from build123d import *

# Parameters (mm, degrees)
PAD021_DEPTH                  = 40.5
POCKET064_DEPTH               = 6
PAD021_MIRRORED041_2_DEPTH    = 40.5
POCKET064_MIRRORED041_2_DEPTH = 6
PAD022_DEPTH                  = 2
PAD022_MIRRORED032_2_DEPTH    = 2
POCKET055_DEPTH               = 30.5
PAD018_DEPTH                  = 19.5
PAD018_FACE36_W               = 39
PAD018_FACE36_H               = 1.2
POCKET061_DEPTH               = 0.2
CHAMFER032_SIZE               = 0.5
CHAMFER030_SIZE               = 1
CHAMFER027_SIZE               = 0.2999
POCKET058_DEPTH               = 10
SKETCH064_W                   = 9.4
SKETCH064_H                   = 50
POCKET070_DEPTH               = 15
POCKET059_DEPTH               = 5
POCKET069_DEPTH               = 10
POCKET062_DEPTH               = 10
POCKET051_DEPTH               = 10
POCKET067_DEPTH               = 10
POCKET054_DEPTH               = 10


with BuildPart() as part:
    # Sketch081 (on DatumPlane) → Pad021 (new body)
    with BuildSketch(Plane.XY.offset(50)):
        with BuildLine():
            ThreePointArc((-47.2, 27.2), (-50.735534, 25.735534), (-52.2, 22.2))
            Line((-52.2, 0), (-52.2, 22.2))
            Line((-50.2, 0), (-52.2, 0))
            Line((-50.2, 22.2), (-50.2, 0))
            ThreePointArc((-47.2, 25.2), (-49.32132, 24.32132), (-50.2, 22.2))
            Line((0, 25.2), (-47.2, 25.2))
            Line((0, 27.2), (0, 25.2))
            Line((-47.2, 27.2), (0, 27.2))
        make_face()
    pad021 = extrude(amount=-PAD021_DEPTH)

    # Sketch080 (on Face10 of Pad021) → Pocket064 (cut)
    with BuildSketch(Plane(origin=(0, 0, 9.5), x_dir=(1, 0, 0), z_dir=(0, 0, -1))):
        with BuildLine():
            ThreePointArc((-50.2, -22.2), (-49.32132, -24.32132), (-47.2, -25.2))
            Line((-47.2, -25.2), (0, -25.2))
            Line((0, -25.2), (0, -26.3))
            Line((0, -26.3), (-47.2, -26.3))
            ThreePointArc((-51.3, -22.2), (-50.099138, -25.099138), (-47.2, -26.3))
            Line((-51.3, 0), (-51.3, -22.2))
            Line((-50.2, 0), (-51.3, 0))
            Line((-50.2, -22.2), (-50.2, 0))
        make_face()
    pocket064 = extrude(amount=-POCKET064_DEPTH, mode=Mode.SUBTRACT)

    # Sketch081 Mirrored041 2 → Pad021 Mirrored041 2 (add)
    with BuildSketch(Plane(origin=(0, 0, 50), x_dir=(-1, 0, 0), z_dir=(0, 0, -1))):
        with BuildLine():
            ThreePointArc((-47.2, 27.2), (-50.735534, 25.735534), (-52.2, 22.2))
            Line((-52.2, 0), (-52.2, 22.2))
            Line((-50.2, 0), (-52.2, 0))
            Line((-50.2, 22.2), (-50.2, 0))
            ThreePointArc((-47.2, 25.2), (-49.32132, 24.32132), (-50.2, 22.2))
            Line((0, 25.2), (-47.2, 25.2))
            Line((0, 27.2), (0, 25.2))
            Line((-47.2, 27.2), (0, 27.2))
        make_face()
    pad021_mirrored041_2 = extrude(amount=PAD021_MIRRORED041_2_DEPTH)

    # Sketch080 Mirrored041 2 → Pocket064 Mirrored041 2 (cut)
    with BuildSketch(Plane(origin=(0, 0, 9.5), x_dir=(-1, 0, 0), z_dir=(0, 0, 1))):
        with BuildLine():
            ThreePointArc((-50.2, -22.2), (-49.32132, -24.32132), (-47.2, -25.2))
            Line((-47.2, -25.2), (0, -25.2))
            Line((0, -25.2), (0, -26.3))
            Line((0, -26.3), (-47.2, -26.3))
            ThreePointArc((-51.3, -22.2), (-50.099138, -25.099138), (-47.2, -26.3))
            Line((-51.3, 0), (-51.3, -22.2))
            Line((-50.2, 0), (-51.3, 0))
            Line((-50.2, -22.2), (-50.2, 0))
        make_face()
    pocket064_mirrored041_2 = extrude(amount=POCKET064_MIRRORED041_2_DEPTH, mode=Mode.SUBTRACT)

    # Mirrored036: Pad021, Pocket064, Pad021 Mirrored041 2, Pocket064 Mirrored041 2 across Sketch081 H_Axis
    add(pad021.mirror(Plane(origin=(0, 0, 50), x_dir=(0, 0, 1), z_dir=(0, 1, 0))))
    add(pocket064.mirror(Plane(origin=(0, 0, 50), x_dir=(0, 0, 1), z_dir=(0, 1, 0))), mode=Mode.SUBTRACT)
    add(pad021_mirrored041_2.mirror(Plane(origin=(0, 0, 50), x_dir=(0, 0, 1), z_dir=(0, 1, 0))))
    add(pocket064_mirrored041_2.mirror(Plane(origin=(0, 0, 50), x_dir=(0, 0, 1), z_dir=(0, 1, 0))), mode=Mode.SUBTRACT)

    # Sketch058 (on DatumPlane) → Pad022 (join)
    with BuildSketch(Plane.XY.offset(50)):
        with BuildLine():
            ThreePointArc((-47.2, 25.2), (-49.32132, 24.32132), (-50.2, 22.2))
            Line((-50.2, 22.2), (-50.2, 0))
            Line((-50.2, 0), (0, 0))
            Line((0, 0), (0, 25.2))
            Line((0, 25.2), (-47.2, 25.2))
        make_face()
    pad022 = extrude(amount=-PAD022_DEPTH)

    # Sketch058 Mirrored032 2 → Pad022 Mirrored032 2 (add)
    with BuildSketch(Plane(origin=(0, 0, 50), x_dir=(-1, 0, 0), z_dir=(0, 0, -1))):
        with BuildLine():
            ThreePointArc((-47.2, 25.2), (-49.32132, 24.32132), (-50.2, 22.2))
            Line((-50.2, 22.2), (-50.2, 0))
            Line((-50.2, 0), (0, 0))
            Line((0, 0), (0, 25.2))
            Line((0, 25.2), (-47.2, 25.2))
        make_face()
    pad022_mirrored032_2 = extrude(amount=PAD022_MIRRORED032_2_DEPTH)

    # Mirrored039: Pad022, Pad022 Mirrored032 2 across Sketch058 H_Axis
    add(pad022.mirror(Plane(origin=(0, 0, 50), x_dir=(0, 0, 1), z_dir=(0, 1, 0))))
    add(pad022_mirrored032_2.mirror(Plane(origin=(0, 0, 50), x_dir=(0, 0, 1), z_dir=(0, 1, 0))))

    # Sketch067 → Pocket055 (cut, symmetric)
    with BuildSketch(Plane.YZ):
        with BuildLine():
            ThreePointArc((-26.1, 12.9), (-26.7, 12.3), (-26.1, 11.7))
            Line((-26.1, 12.9), (-26.1, 11.7))
        make_face()
    pocket055 = extrude(amount=POCKET055_DEPTH, both=True, mode=Mode.SUBTRACT)

    # Sketch067 → Pad018 (join, symmetric)
    with BuildSketch(Plane.YZ):
        with BuildLine():
            ThreePointArc((-26.1, 12.9), (-26.7, 12.3), (-26.1, 11.7))
            Line((-26.1, 12.9), (-26.1, 11.7))
        make_face()
    pad018 = extrude(amount=PAD018_DEPTH, both=True)

    # Pad018 Face36 → Pocket061 (cut)
    with BuildSketch(Plane(origin=(0, -26.1, 12.3), x_dir=(1, 0, 0), z_dir=(0, 1, 0))):
        Rectangle(PAD018_FACE36_W, PAD018_FACE36_H)
    pocket061 = extrude(amount=-POCKET061_DEPTH, mode=Mode.SUBTRACT)

    # Mirrored040: Pocket055, Pad018, Pocket061 across Sketch067 V_Axis
    add(pocket055.mirror(Plane(origin=(0, 0, 0), x_dir=(1, 0, 0), z_dir=(0, 1, 0))), mode=Mode.SUBTRACT)
    add(pad018.mirror(Plane(origin=(0, 0, 0), x_dir=(1, 0, 0), z_dir=(0, 1, 0))))
    add(pocket061.mirror(Plane(origin=(0, 0, 0), x_dir=(1, 0, 0), z_dir=(0, 1, 0))), mode=Mode.SUBTRACT)

    # Chamfer032
    chamfer032_edges = [part.edges().sort_by_distance(p)[0] for p in [
        (0, -27.2, 9.5),
    ]]
    chamfer(chamfer032_edges, length=CHAMFER032_SIZE)

    # Chamfer030
    chamfer030_edges = [part.edges().sort_by_distance(p)[0] for p in [
        (0, -27.2, 50),
    ]]
    chamfer(chamfer030_edges, length=CHAMFER030_SIZE)

    # Chamfer027
    chamfer027_edges = [part.edges().sort_by_distance(p)[0] for p in [
        (50.2, 0, 48),
    ]]
    chamfer(chamfer027_edges, length=CHAMFER027_SIZE)

    # Sketch079 (on DatumPlane) → Pocket058 (cut)
    with BuildSketch(Plane.YZ.offset(52.2)):
        Polygon((-7.2, 7.6), (-7.2, 15.6), (-12.1, 15.6), (-12.1, 18.1), (-14.1, 18.1), (-14.1, 15.6), (-17.8, 15.6), (-17.8, 7.6), (-17.8, 2.6), (-7.2, 2.6), align=None)
    extrude(amount=-POCKET058_DEPTH, mode=Mode.SUBTRACT)

    # Sketch064 (on DatumPlane) → Pocket070 (cut)
    with BuildSketch(Plane.YZ.offset(52.2)):
        with Locations((0, -6)):
            Rectangle(SKETCH064_W, SKETCH064_H)
    extrude(amount=-POCKET070_DEPTH, mode=Mode.SUBTRACT)

    # Sketch065 (on DatumPlane) → Pocket059 (cut)
    with BuildSketch(Plane.YZ.offset(52.2)):
        with BuildLine():
            Line((7.9, -40.25), (7.9, 9.75))
            ThreePointArc((9.15, 11), (8.266117, 10.633883), (7.9, 9.75))
            Line((9.15, 11), (15.85, 11))
            ThreePointArc((17.1, 9.75), (16.733883, 10.633883), (15.85, 11))
            Line((17.1, 9.75), (17.1, -40.25))
            Line((7.9, -40.25), (17.1, -40.25))
        make_face()
    extrude(amount=-POCKET059_DEPTH, mode=Mode.SUBTRACT)

    # Sketch078 (on DatumPlane) → Pocket069 (cut)
    with BuildSketch(Plane(origin=(-52.2, 0, 0), x_dir=(0, -1, 0), z_dir=(-1, 0, 0))):
        Polygon((-15.02, 7.6), (-15.02, 15.6), (-20.32, 15.6), (-20.32, 18.1), (-22.32, 18.1), (-22.32, 15.6), (-25.62, 15.6), (-25.62, 7.6), (-25.62, -42.4), (-15.02, -42.4), align=None)
    extrude(amount=-POCKET069_DEPTH, mode=Mode.SUBTRACT)

    # Sketch075 (on DatumPlane) → Pocket062 (cut)
    with BuildSketch(Plane(origin=(-52.2, 0, 0), x_dir=(0, -1, 0), z_dir=(-1, 0, 0))):
        Polygon((-4.86, 7.6), (-4.86, 15.6), (-10.16, 15.6), (-10.16, 18.1), (-12.16, 18.1), (-12.16, 15.6), (-15.46, 15.6), (-15.46, 7.6), (-15.46, -42.4), (-4.86, -42.4), align=None)
    extrude(amount=-POCKET062_DEPTH, mode=Mode.SUBTRACT)

    # Sketch073 (on DatumPlane) → Pocket051 (cut)
    with BuildSketch(Plane(origin=(-52.2, 0, 0), x_dir=(0, -1, 0), z_dir=(-1, 0, 0))):
        Polygon((5.3, 7.6), (5.3, 15.6), (0, 15.6), (0, 18.1), (-2, 18.1), (-2, 15.6), (-5.3, 15.6), (-5.3, 7.6), (-5.3, -42.4), (5.3, -42.4), align=None)
    extrude(amount=-POCKET051_DEPTH, mode=Mode.SUBTRACT)

    # Sketch077 (on DatumPlane) → Pocket067 (cut)
    with BuildSketch(Plane(origin=(-52.2, 0, 0), x_dir=(0, -1, 0), z_dir=(-1, 0, 0))):
        Polygon((15.46, 7.6), (15.46, 15.6), (10.16, 15.6), (10.16, 18.1), (8.16, 18.1), (8.16, 15.6), (4.86, 15.6), (4.86, 7.6), (4.86, -42.4), (15.46, -42.4), align=None)
    extrude(amount=-POCKET067_DEPTH, mode=Mode.SUBTRACT)

    # Sketch066 (on DatumPlane) → Pocket054 (cut)
    with BuildSketch(Plane(origin=(-52.2, 0, 0), x_dir=(0, -1, 0), z_dir=(-1, 0, 0))):
        Polygon((25.62, 7.6), (25.62, 15.6), (20.32, 15.6), (20.32, 18.1), (18.32, 18.1), (18.32, 15.6), (15.02, 15.6), (15.02, 7.6), (15.02, -42.4), (25.62, -42.4), align=None)
    extrude(amount=-POCKET054_DEPTH, mode=Mode.SUBTRACT)


solid = part.part
Can you work these out from the model? Positions are in its coordinate system, mm. A direction names the side the tool comes from. Give positions to 0.01 mm unless a question says otherwise; leave off trailing zeros. Loops run counter-clockwise (first coordinate to the right, second up) from the corner with the lowest first, then second, coordinate; pieces in that order, holes last. Notation, with made-up numbers: M 16.5,87 L 62.5,87 A18 cw 62.5,112 Z; hole C 89,59 d9. An arc over 180 degrees is marked long. One line per item, written item: value.
1) I'm going to push flat-ended pins straight in: pin 1 (12 mm diameter, centred on x = 10.5, y = -11, fed in from -Z); pin 2 (3 mm diameter, centred on y = -5.5, z = 12.5, fed in from -X); pin 3 (1 mm diameter, centred on x = 51.5, y = -0.5, fed in from -Z). Where does each tip first touch, or does it pass through?
Geometry check:
pin 1: stops at z = 48
pin 2: stops at x = 51.3
pin 3: stops at z = 19
2) Please list where these lines run through material, in increasing order: line 1 (X direction, y = -9, z = 46); line 2 (Y direction, x = -43, z = 21); line 3 (Z direction, x = 25, y = 11).
Geometry check:
line 1: x = -52.2 to -50.2, 50.2 to 52.2
line 2: y = -27.2 to -25.2, 25.2 to 27.2
line 3: z = 48 to 50
3) Thinking about a two-plate mould opening in X: for faces 6 (the face through (1, 0, 50)), 7 (the face through (50.446, -25.519, 9.642)), 8 (the face through (49.212, 24.168, 47.885)), which applies, +X half, -X half, draft (parallel to the pull), parting line (faces both ways), or undercut?
Geometry check:
face 6: draft
face 7: +X half
face 8: undercut
4) Imagine slicing it at D-D on x = -29.5. Write out the boundary of the cut face in (y, z), and give its area (3 significant figures).
Geometry check:
outline: M -27.2,10 L -26.7,9.5 L -26.3,9.5 L -26.3,11.73 A0.6 cw -26.3,12.87 L -26.3,15.5 L -25.2,15.5 L -25.2,47.7 L -24.9,48 L 24.9,48 L 25.2,47.7 L 25.2,15.5 L 26.3,15.5 L 26.3,12.87 A0.6 cw 26.3,11.73 L 26.3,9.5 L 26.7,9.5 L 27.2,10 L 27.2,49 L 26.2,50 L -26.2,50 L -27.2,49 Z
area: 248 mm²
5) Imagine slicing it at C-C on z = 17. Count the separate pieces of the cut face and the enclosed holes in it, and give its area (3 significant figures).
Geometry check:
separate pieces: 7
enclosed holes: 0
area: 563 mm²
6) Imagine slicing it at A-A on z = 29.5. Write out the boundary of the cut face in (x, y), and give its area (3 significant figures).
Geometry check:
outline: M -52.2,-22.2 A5 ccw -47.2,-27.2 L 47.2,-27.2 A5 ccw 52.2,-22.2 L 52.2,22.2 A5 ccw 47.2,27.2 L -47.2,27.2 A5 ccw -52.2,22.2 Z; hole M -50.2,-22.2 A3 ccw -47.2,-25.2 L 47.2,-25.2 A3 ccw 50.2,-22.2 L 50.2,22.2 A3 ccw 47.2,25.2 L -47.2,25.2 A3 ccw -50.2,22.2 Z
area: 605 mm²
7) Imagine slicing it at B-B on x = -44. Write out the boundary of the cut face in (y, z), and give its area (3 significant figures).
Geometry check:
outline: M -27.2,10 L -26.7,9.5 L -26.3,9.5 L -26.3,15.5 L -25.62,15.5 L -25.62,15.6 L -25.2,15.6 L -25.2,47.7 L -24.9,48 L 24.9,48 L 25.2,47.7 L 25.2,15.6 L 25.62,15.6 L 25.62,15.5 L 26.3,15.5 L 26.3,9.5 L 26.7,9.5 L 27.2,10 L 27.2,49 L 26.2,50 L -26.2,50 L -27.2,49 Z
area: 248 mm²
8) On a 3-axis mill with a long thin cutter (end or side, diameter ignored), from which of +Z, -Z, +X, -X, +Y, -Y can I reach the whole of each face in a straight line? I mean faces 1 (the face through (52, -4.7, 15)), 2 (the face through (-50.7, 25.77, 29.77)), 3 (the face through (52, -17.8, 13)), 4 (the face through (-51, -9, 18.1)), 5 (the face through (-48.4, -26.12, 12.46)). Say none if no direction works.
Geometry check:
face 1: -Z, +X
face 2: +Z, -Z, -X, +Y
face 3: -Z, +X, -X
face 4: -Z, -X
face 5: -Z
